Autodesk Inventor part; units mm, degrees
ref_plane "Work Plane1" through (3.5, 0, 0) normal (0, 0, 1) x (1, 0, 0)
ref_plane "YZ Plane" through (0, 0, 0) normal (1, 0, 0) x (0, 1, 0)
ref_plane "XZ Plane" through (0, 0, 0) normal (0, 1, 0) x (-1, 0, 0)
sketch "Sketch1" plane through (0, 0, 0) normal (0, 0, 1) x (1, 0, 0)
  line L0 (0, 5) -> (0, 2.0092)
  line L1 (1.6, 2.5) -> (16, 2.5)
  line L2 (16, 2.5) -> (16, 0)
  line L3 (16, 0) -> (-0.86, 0)
  line L4 (0, -1) -> (0, 6)
  line L5 (-4.232, 0) -> (19.372, 0)
  line L6 (-0.86, 0) -> (-0.86, 5)
  line L7 (-0.86, 5) -> (0, 5)
  line L8 (1.6, 2.5) -> (1.1092, 2.0092)
  line L9 (1.1092, 2.0092) -> (0, 2.0092)
  dimension "d0" = 16
  dimension "d1" = 14.4
  dimension "d2" = 5
  dimension "d8" = 0.86
  dimension "d9" = 10
  dimension "d15" = 4.0185
  dimension "d16" = 0.4908
revolve "Body" add sketch "Sketch1" angle 360 about axis through (16, 0, 0) along (-1, 0, 0)
sketch "Sketch2" plane through (0, 0, 0) normal (1, 0, 0) x (0, 0, -1)
  circle A0 centre (0, 0) radius 5
  line L0 (0, 4.0415) -> (3.5, 2.0207)
  line L1 (3.5, 2.0207) -> (3.5, -2.0207)
  line L2 (3.5, -2.0207) -> (0, -4.0415)
  line L3 (0, -4.0415) -> (-3.5, -2.0207)
  line L4 (-3.5, -2.0207) -> (-3.5, 2.0207)
  line L5 (-3.5, 2.0207) -> (0, 4.0415)
  circle A1 centre (0, 0) radius 5
  dimension "d10" = 7
extrude "Head" add sketch "Sketch2" against normal blind 4.51 contours L0 L1 L2 L3 L4 L5
sketch "Sketch3" plane through (0, 0, 0) normal (0, 0, 1) x (1, 0, 0)
  line L0 (-4.51, 3.15) -> (-4.51, 4.0415)
  line L1 (-4.51, 4.0415) -> (-3.9953, 4.0415)
  line L2 (-3.9953, 4.0415) -> (-4.51, 3.15)
  line L3 (-2.0945, 4.0415) -> (-4.51, 4.0415)
  line L4 (-4.51, 4.0415) -> (-4.51, 1.7321)
  line L5 (-0.86, 4.0415) -> (-4.51, 4.0415)
  line L6 (-4.51, 4.0415) -> (-4.51, 2.0207)
  line L7 (-5.24, 0) -> (-0.13, 0)
  dimension "d5" = 30
  dimension "d18" = 6.3
revolve "Chamfer1" cut sketch "Sketch3" angle 360 about axis through (-10, 0, 0) along (1, 0, 0)
thread "Thread"
chamfer "Chamfer2" distance 0.4908 distance2 0.4908 1 edges at (16, -2.5, 0) measured on face at (16, 0.6587, 0.3326)
ref_plane "Work Plane1" through (3.5, 0, 0) normal (0, 0, 1) x (1, 0, 0)
equation "\"d10\" = SW"
equation "\"d3\" = KOH"
equation "\"d13\" = GEL"
equation "\"d6\" = -0.5 * SPD + 0.5 * GD"
equation "\"d7\" = -0.5 * SPD + 0.5 * GD"
equation "\"d0\" = NLG"
equation "\"d1\" = GEL"
equation "\"d2\" = GD"
equation "\"d8\" = PHH"
equation "\"d9\" = LADI"
equation "\"d15\" = BDM"
equation "\"d16\" = GAL"
equation "\"d5\" = ANG1"
equation "\"d18\" = SW0"
equation "\"NLG\" = 16"
equation "\"GD\" = NND"
equation "\"BDM\" = NND - 1.2269 * PTC"
equation "\"KOH\" = 4.51"
equation "\"GEL\" = 14.4"
equation "\"LADI\" = 10"
equation "\"SW\" = 7"
equation "\"PHH\" = 0.86"
equation "\"SW0\" = 6.3"
equation "\"SPD\" = NND - 1.2269 * PTC"
equation "\"ANG1\" = 30deg"
equation "\"GAL\" = 0.61345 * PTC"
equation "\"GUL\" = 0.61345 * PTC"
equation "\"WFT\" = PHH"
equation "\"PTC\" = 0.8"
equation "\"THREADDIA\" = 5"
equation "\"E0\" = 1.155 * SW"
equation "\"TOA\" = 30deg"
equation "\"NND\" = 5"
equation "\"GD1\" = THREADDIA - 1.2269 * PTC"
equation "\"SDH\" = 5.7"
equation "\"KOH1\" = 3.65"
equation "\"SD2\" = NND"
equation "\"SD\" = 0"
equation "\"RR\" = 0.2"
properties part number "AS 1427 - M5 x 16" material "Steel, Mild"
For this review, take the finished solid that the model builds, in its own axes (mm). A direction names the side the tool comes from. Coordinates: 2 decimals unless noted, no trailing zeros. Write each loop counter-clockwise with the first axis right and the second up, starting at its lowest first coordinate (ties: lowest second). Pieces come first, ordered by that corner, then holes. Notation, with made-up numbers: (-13.5, 25.25) -> (4.5, 25.25) arc R19 ccw to (4.5, 30.25) -> close; hole circle Ø1 at (35.25, 58.25). An arc over 180 degrees is marked (long way). Put each result on its own line as item: value.
Q1. Take a section at A-A, the plane y = 0. State the section outline as (x, z) points.
From the geometry:
outline: (-4.51, -3.15) -> (-4.31, -3.5) -> (-0.86, -3.5) -> (-0.86, -5) -> (0, -5) -> (0, -2.01) -> (1.11, -2.01) -> (1.6, -2.5) -> (15.51, -2.5) -> (16, -2.01) -> (16, 2.01) -> (15.51, 2.5) -> (1.6, 2.5) -> (1.11, 2.01) -> (0, 2.01) -> (0, 5) -> (-0.86, 5) -> (-0.86, 3.5) -> (-4.31, 3.5) -> (-4.51, 3.15) -> close
Q2. Tool access review of faces 4 (the flat face through (-2.6, 3, 1.8)), 5 (the flat face through (0, 2.2, -0.1)), 6 (the flat face through (-2.56, 3.045, -1.726)), 7 (the flat face through (-3, 0, 3.5)), 8 (the flat face through (-0.86, 0, 4)): name each direction out of +Z, -Z, +X, -X, +Y, -Y from which nothing blocks a thin tool from reaching the whole face with its end or side.
From the geometry:
face 4: +Z, -X, +Y
face 5: none
face 6: -Z, -X, +Y
face 7: +Z, -X, +Y, -Y
face 8: -X
Q3. Clearance check with flat-ended pins moving along their axes: pin 1 Ø3 at (x, z) = (9, 2) entering from -Y; pin 2 Ø6 at (x, y) = (13, 1) entering from +Z; pin 3 Ø1 at (x, y) = (-2, 0) entering from +Z. State where each tip first meets the part, or that it passes through.
From the geometry:
pin 1: stops at y = -2.45
pin 2: stops at z = 2.5
pin 3: stops at z = 3.5
Q4. Take a section at B-B, the plane x = -2. State the section outline as (y, z) points.
From the geometry:
outline: (-4.04, 0) -> (-2.02, -3.5) -> (2.02, -3.5) -> (4.04, 0) -> (2.02, 3.5) -> (-2.02, 3.5) -> close
Q5. Wall thickness on L1, parallel to Z at x = 10, y = 0; L2, parallel to X at y = -0.25, z = 4.25; L3, parallel to Z at x = 1.75, y = 1.5: over which ranges is each line inside the solid? List them lowest first.
From the geometry:
L1: z = -2.5 to 2.5
L2: x = -0.86 to 0
L3: z = -2 to 2
Q6. Take a section at C-C, the plane x = 5. State the section outline as (y, z) points.
From the geometry:
outline: circle Ø5 at (0, 0)
Q7. The part is to be moulded in two halves that separate along X. For faces 1 (the flat face through (-3, 0, -3.5)), 2 (the flat face through (16, 0, 0)), 3 (the cylindrical face through (0.547, 1.916, -0.604)), say which applies: +X half, -X half, draft (parallel to the pull), parting line (faces both ways), or undercut.
From the geometry:
face 1: draft
face 2: +X half
face 3: undercut
